Work out the finished part from the listing and answer in its coordinate system (mm). A direction names the side the tool comes from. Coordinates: 2 decimals unless noted, no trailing zeros. Loops run counter-clockwise (first coordinate to the right, second up) from the corner with the lowest first, then second, coordinate; pieces in that order, holes last.
```python
from build123d import *

# Parameters (mm, degrees)
SKETCH2_W           = 24.765
SKETCH2_H           = 15.875
BOSS_EXTRUDE1_DEPTH = 19.05
SKETCH3_W           = 28.575
SKETCH3_H           = 22.86
BOSS_EXTRUDE2_DEPTH = 38.1
SKETCH4_W           = 6.35
SKETCH4_H           = 23.8125
SKETCH4_W_2         = 11.049
CUT_EXTRUDE1_DEPTH  = 47.6725
FILLET5_R           = 11.43
SKETCH7_R           = 6.477
CUT_EXTRUDE3_DEPTH  = 46.56539833
FILLET3_R           = 6.35
BOSS_EXTRU_1_REACH  = 50.977
CONG_3_R            = 4


with BuildPart() as part:
    # Sketch2 → Boss-Extrude1 (new body)
    with BuildSketch(Plane.XY):
        Rectangle(SKETCH2_W, SKETCH2_H)
    extrude(amount=-BOSS_EXTRUDE1_DEPTH)

    # Sketch3 → Boss-Extrude2 (add)
    with BuildSketch(Plane.XY):
        Rectangle(SKETCH3_W, SKETCH3_H)
    extrude(amount=BOSS_EXTRUDE2_DEPTH)

    # Sketch4 → Cut-Extrude1 (cut, through all)
    with BuildSketch(Plane(origin=(0, -11.43, 0), x_dir=(-1, 0, 0), z_dir=(0, -1, 0))):
        with Locations((11.1125, -26.19375)):
            Rectangle(SKETCH4_W, SKETCH4_H)
        with Locations((-3.175, -26.19375)):
            Rectangle(SKETCH4_W_2, SKETCH4_H)
    extrude(amount=-CUT_EXTRUDE1_DEPTH, mode=Mode.SUBTRACT)

    # Fillet5
    fillet5_edges = [part.edges().sort_by_distance(p)[0] for p in [
        (-5.1435, -11.43, 38.1),
        (-5.1435, 11.43, 38.1),
        (11.4935, 11.43, 38.1),
        (11.4935, -11.43, 38.1),
    ]]
    fillet(fillet5_edges, radius=FILLET5_R - 0.0001)  # a hair under: the kernel refuses the full size

    # Sketch7 → Cut-Extrude3 (cut, through all)
    with BuildSketch(Plane.ZY.offset(7.9375)):
        with Locations(Location((26.67, 0, 0), (0, 0, 270))):
            Circle(SKETCH7_R)
    extrude(amount=-CUT_EXTRUDE3_DEPTH, mode=Mode.SUBTRACT)

    # Fillet3
    fillet3_edges = [part.edges().sort_by_distance(p)[0] for p in [
        (-12.3825, 7.9375, -9.525),
        (12.3825, 7.9375, -9.525),
        (12.3825, -7.9375, -9.525),
        (-12.3825, -7.9375, -9.525),
    ]]
    fillet(fillet3_edges, radius=FILLET3_R)

    # Boss.-Extru.1: up to this face of the body (flat: up to its plane)
    boss_extru_1_end = Plane(part.part.faces().sort_by_distance((14.2875, 0, 16.22567269))[0])
    # Esquisse1 → Boss.-Extru.1 (add, up to the picked face)
    with BuildSketch(Plane.ZY.offset(14.2875), mode=Mode.PRIVATE) as boss_extru_1_sk1:
        Polygon((14.2875, 11.43), (17.927202343, 11.43), (14.2875, 1.43), align=None)
    boss_extru_1_tool1 = split(extrude(boss_extru_1_sk1.sketch, amount=-BOSS_EXTRU_1_REACH, mode=Mode.PRIVATE), bisect_by=boss_extru_1_end, keep=Keep.BOTH, mode=Mode.PRIVATE)
    boss_extru_1 = boss_extru_1_tool1.solids().sort_by(Axis((-14.2875, 8.096667, 15.500734), (1, 0, 0)))[0]
    add(boss_extru_1)

    # Symétrie1: Boss.-Extru.1 across plane
    add(boss_extru_1.mirror(Plane.ZX))

    # Congé3
    cong_3_edges = [part.edges().sort_by_distance(p)[0] for p in [
        (-11.1125, 1.43, 14.2875),
        (3.175, 1.43, 14.2875),
        (-11.1125, -1.43, 14.2875),
        (3.175, -1.43, 14.2875),
    ]]
    fillet(cong_3_edges, radius=CONG_3_R)


solid = part.part
```
1. Each of these flat-tipped pins is pushed along its axis until it touches: P1, Ø2, axis at x = 0.5, y = -1.5, coming from the +Z side; P2, Ø1, axis at x = 8, z = -2, coming from the +Y side; P3, Ø9.5, axis at x = 2, z = -12.5, coming from the -Y side; P4, Ø8, axis at y = 0, z = 26.67, coming from the -X side. Where does it stop, or does it pass through?
2. Straight lines are drawn through the part: probe 1 along Z at (x, y) = (-4.5, 0); probe 2 along X at (y, z) = (-3.5, 35); probe 3 along Y at (x, z) = (-3, -6). For each, find the intervals that lie inside material, in ascending order.
3. For faces 4 (the cylindrical face through (3.252, -1.41, 14.347)), 5 (the flat face through (-12.382, 0, -9)), 6 (the flat face through (-11, 0, 14.288)), 7 (the cylindrical face through (10.6, 6, -9.7)), determine the directions among +Z, -Z, +X, -X, +Y, -Y from which every point of the face is accessible in a straight line to the end or side of a thin tool.
4. A cutting plane is placed at C-C, the plane y = -5. Give the vertices of the cut face in (x, z).
5. A cutting plane is placed at B-B, the plane z = -7. Give the vertices of the cut face in (x, y).
6. A cutting plane is placed at D-D, the plane x = -0.5. Give the vertices of the cut face in (y, z).
7. Determine the mould class of faces 1 (the cylindrical face through (-5.104, 8.171, 34.663)), 2 (the flat face through (0, 0, -19.05)), 3 (the cylindrical face through (-5.183, 1.404, 20.347)) for opening direction Y: released by +Y, released by -Y, zero draft, split by the parting line, or undercut.
Answers below:
1. P1: stops at z = 14.68
1. P2: stops at y = 7.77
1. P3: stops at y = -7.94
1. P4: passes through
2. probe 1: z = -19.05 to 20.19, 33.15 to 38.1
2. probe 2: x = -7.94 to -2.35, 8.7 to 14.29
2. probe 3: y = -7.94 to 7.94
3. face 4: +Z
3. face 5: -Z, -X, +Y, -Y
3. face 6: +Z, -X
3. face 7: -Z, +X, +Y
4. outline: (-14.29, 0) - (-11.39, 0) - (-11.39, -19.05) - (11.39, -19.05) - (11.39, 0) - (14.29, 0) - (14.29, 22.55) - (8.7, 22.55) - (8.7, 15.59) - (-2.35, 15.59) - (-2.35, 22.55) - (-7.94, 22.55) - (-7.94, 15.59) - (-14.29, 15.59) - close; (-7.94, 30.79) - (-2.35, 30.79) - (-2.35, 36.95) - (-7.94, 36.95) - close; (8.7, 30.79) - (14.29, 30.79) - (14.29, 36.95) - (8.7, 36.95) - close
5. outline: (-12.38, -1.59) arc R6.35 ccw to (-6.03, -7.94) - (6.03, -7.94) arc R6.35 ccw to (12.38, -1.59) - (12.38, 1.59) arc R6.35 ccw to (6.03, 7.94) - (-6.03, 7.94) arc R6.35 ccw to (-12.38, 1.59) - close
6. outline: (-11.43, 0) - (-7.94, 0) - (-7.94, -19.05) - (7.94, -19.05) - (7.94, 0) - (11.43, 0) - (11.43, 17.93) - (2.09, 14.53) arc R4 cw to (0.72, 14.29) - (-0.72, 14.29) arc R4 cw to (-2.09, 14.53) - (-11.43, 17.93) - close
7. face 1: released by +Y
7. face 2: zero draft
7. face 3: undercut
